```python
from build123d import *

# Parameters (mm, degrees)
SKETCH1_W                      = 172.4
SKETCH1_H                      = 192.4
BOSS_EXTRUDE1_DEPTH            = 6.35
CUT_EXTRUDE1_REACH             = 131.326
SKETCH2_W                      = 41
SKETCH2_H                      = 41
CBORE_FOR_M4_SHCS1_D           = 4.5
CBORE_FOR_M4_SHCS1_CBORE_D     = 8
CBORE_FOR_M4_SHCS1_CBORE_DEPTH = 4
CUT_EXTRUDE3_REACH             = 131.326
SKETCH5_R                      = 1.2
SKETCH6_R                      = 1.4
CUT_EXTRUDE4_DEPTH             = 4
CUT_EXTRUDE5_REACH             = 131.326
SKETCH7_R                      = 1.35
SKETCH8_R                      = 1.5
CUT_EXTRUDE6_DEPTH             = 5
SKETCH9_W                      = 3
SKETCH9_H                      = 192.4
EXTRUDE_THIN1_DEPTH            = 3
CHAMFER1_SIZE                  = 3
CHAMFER2_SIZE                  = 1
CUT_EXTRUDE8_DEPTH             = 302.265202936
CUT_EXTRUDE8_DEPTH_BACK        = 302.265202936
SKETCH11_W                     = 285.28996188
SKETCH11_H                     = 259.000443209
SKETCH11_W_2                   = 75.460655446
SKETCH11_H_2                   = 65.723796679


with BuildPart() as part:
    # Sketch1 → Boss-Extrude1 (new body)
    with BuildSketch(Plane(origin=(0, 0, 0), x_dir=(1, 0, 0), z_dir=(0, 1, 0))):
        Rectangle(SKETCH1_W, SKETCH1_H)
    extrude(amount=BOSS_EXTRUDE1_DEPTH)

    # Sketch2 → Cut-Extrude1 (cut, up to next)
    with BuildSketch(Plane(origin=(0, 6.35, 0), x_dir=(1, 0, 0), z_dir=(0, 1, 0)), mode=Mode.PRIVATE) as cut_extrude1_sk1:
        with Locations((-65.7, 75.7)):
            Rectangle(SKETCH2_W, SKETCH2_H)
    cut_extrude1_tool1 = extrude(cut_extrude1_sk1.sketch, amount=-CUT_EXTRUDE1_REACH, mode=Mode.PRIVATE) & part.part
    add(cut_extrude1_tool1.solids().sort_by_distance((-65.7, 6.35, -75.7))[0], mode=Mode.SUBTRACT)

    # CBORE for M4 SHCS1 (through all)
    with Locations(Plane(origin=(0, 6.35, 0), x_dir=(1, 0, 0), z_dir=(0, 1, 0))):
        with Locations((66.2, 76.2), (-66.2, 34.39549116), (-66.2, -56.2), (-26.2, 76.2)):
            CounterBoreHole(CBORE_FOR_M4_SHCS1_D / 2, CBORE_FOR_M4_SHCS1_CBORE_D / 2, CBORE_FOR_M4_SHCS1_CBORE_DEPTH)

    # Sketch5 → Cut-Extrude3 (cut, up to next)
    with BuildSketch(Plane(origin=(0, 6.35, 0), x_dir=(1, 0, 0), z_dir=(0, 1, 0)), mode=Mode.PRIVATE) as cut_extrude3_sk1:
        with Locations(Location((-76.36, -87.31, 0), (0, 0, 270))):
            Circle(SKETCH5_R)
    cut_extrude3_tool1 = extrude(cut_extrude3_sk1.sketch, amount=-CUT_EXTRUDE3_REACH, mode=Mode.PRIVATE) & part.part
    # Sketch5 → Cut-Extrude3 (cut, up to next)
    with BuildSketch(Plane(origin=(0, 6.35, 0), x_dir=(1, 0, 0), z_dir=(0, 1, 0)), mode=Mode.PRIVATE) as cut_extrude3_sk2:
        with Locations(Location((-56.04, -87.31, 0), (0, 0, 270))):
            Circle(SKETCH5_R)
    cut_extrude3_tool2 = extrude(cut_extrude3_sk2.sketch, amount=-CUT_EXTRUDE3_REACH, mode=Mode.PRIVATE) & part.part
    add(cut_extrude3_tool1.solids().sort_by_distance((-76.36, 6.35, 87.31))[0], mode=Mode.SUBTRACT)
    add(cut_extrude3_tool2.solids().sort_by_distance((-56.04, 6.35, 87.31))[0], mode=Mode.SUBTRACT)

    # Sketch6 → Cut-Extrude4 (cut)
    with BuildSketch(Plane(origin=(0, 6.35, 0), x_dir=(1, 0, 0), z_dir=(0, 1, 0))):
        with Locations(Location((-76.36, -87.31, 0), (0, 0, 270))):
            Circle(SKETCH6_R)
        with Locations(Location((-56.04, -87.31, 0), (0, 0, 270))):
            Circle(SKETCH6_R)
    extrude(amount=-CUT_EXTRUDE4_DEPTH, mode=Mode.SUBTRACT)

    # Sketch7 → Cut-Extrude5 (cut, up to next)
    with BuildSketch(Plane(origin=(0, 6.35, 0), x_dir=(1, 0, 0), z_dir=(0, 1, 0)), mode=Mode.PRIVATE) as cut_extrude5_sk1:
        with Locations(Location((-35.24, -50.96, 0), (0, 0, 270))):
            Circle(SKETCH7_R)
    cut_extrude5_tool1 = extrude(cut_extrude5_sk1.sketch, amount=-CUT_EXTRUDE5_REACH, mode=Mode.PRIVATE) & part.part
    # Sketch7 → Cut-Extrude5 (cut, up to next)
    with BuildSketch(Plane(origin=(0, 6.35, 0), x_dir=(1, 0, 0), z_dir=(0, 1, 0)), mode=Mode.PRIVATE) as cut_extrude5_sk2:
        with Locations(Location((23.46, -50.96, 0), (0, 0, 270))):
            Circle(SKETCH7_R)
    cut_extrude5_tool2 = extrude(cut_extrude5_sk2.sketch, amount=-CUT_EXTRUDE5_REACH, mode=Mode.PRIVATE) & part.part
    add(cut_extrude5_tool1.solids().sort_by_distance((-35.24, 6.35, 50.96))[0], mode=Mode.SUBTRACT)
    add(cut_extrude5_tool2.solids().sort_by_distance((23.46, 6.35, 50.96))[0], mode=Mode.SUBTRACT)

    # Sketch8 → Cut-Extrude6 (cut)
    with BuildSketch(Plane(origin=(0, 6.35, 0), x_dir=(1, 0, 0), z_dir=(0, 1, 0))):
        with Locations(Location((-35.24, -50.96, 0), (0, 0, 270))):
            Circle(SKETCH8_R)
        with Locations(Location((23.46, -50.96, 0), (0, 0, 270))):
            Circle(SKETCH8_R)
    extrude(amount=-CUT_EXTRUDE6_DEPTH, mode=Mode.SUBTRACT)

    # Sketch9 → Extrude-Thin1 (add)
    with BuildSketch(Plane(origin=(0, 6.35, 0), x_dir=(1, 0, 0), z_dir=(0, 1, 0))):
        with Locations((78.7, 0)):
            Rectangle(SKETCH9_W, SKETCH9_H)
    extrude(amount=EXTRUDE_THIN1_DEPTH)

    # Chamfer1
    chamfer1_edges = [part.edges().sort_by_distance(p)[0] for p in [
        (77.2, 6.35, 0),
        (80.2, 6.35, 0),
    ]]
    chamfer(chamfer1_edges, length=CHAMFER1_SIZE - 0.0001)  # a hair under: the kernel refuses the full size

    # Chamfer2
    chamfer2_edges = [part.edges().sort_by_distance(p)[0] for p in [
        (0, 0, 96.2),
        (86.2, 0, 0),
    ]]
    chamfer(chamfer2_edges, length=CHAMFER2_SIZE)


with BuildPart() as body_2:
    # Mirror1: mirrored copy
    add(part.part.mirror(Plane(origin=(1.506427127, 3.750129783, 96.2), x_dir=(1, 0, 0), z_dir=(0, 0, 1))))

    # Sketch11 → Cut-Extrude8 (cut, two sides: drawn at the far end of the back side and taken through both)
    with BuildSketch(Plane(origin=(0, 6.35, 0), x_dir=(1, 0, 0), z_dir=(0, 1, 0)).offset(-CUT_EXTRUDE8_DEPTH_BACK)):
        with Locations((10.467123175, -184.853934456)):
            Rectangle(SKETCH11_W, SKETCH11_H)
        with Locations((-5.84211526, -117.426187493)):
            Rectangle(SKETCH11_W_2, SKETCH11_H_2, mode=Mode.SUBTRACT)
    extrude(amount=CUT_EXTRUDE8_DEPTH + CUT_EXTRUDE8_DEPTH_BACK, mode=Mode.SUBTRACT)


solid = body_2.part
```
Input: part model. Units: mm. Frame: model coordinates. A direction names the side the tool comes from. Coordinates: 2 decimals unless noted, no trailing zeros. Write each loop counter-clockwise with the first axis right and the second up, starting at its lowest first coordinate (ties: lowest second). Pieces come first, ordered by that corner, then holes. Notation, with made-up numbers: (53, 42.25) -> (92, 42.25) arc R10 cw to (92, 55.25) -> close; hole circle Ø10 at (8.5, -31). An arc over 180 degrees is marked (long way). Write each question's results on one line, items separated by ' | '.
Item 1: Material intervals for probe 1 along X at (y, z) = (4.5, 141.5); probe 2 along Z at (x, y) = (11.5, 0.5), sorted ascending.
Conclusion:
probe 1: x = -43.57 to -36.74, -33.74 to 21.96, 24.96 to 31.89 | probe 2: z = 96.7 to 150.29
Item 2: Section query B-B on z = 141.44. Return loops of the section in (x, y).
Conclusion:
outline: (-43.57, 0) -> (-36.59, 0) -> (-36.59, 1.35) -> (-36.74, 1.35) -> (-36.74, 6.35) -> (-43.57, 6.35) -> close; (-33.89, 0) -> (22.11, 0) -> (22.11, 1.35) -> (21.96, 1.35) -> (21.96, 6.35) -> (-33.74, 6.35) -> (-33.74, 1.35) -> (-33.89, 1.35) -> close; (24.81, 0) -> (31.89, 0) -> (31.89, 6.35) -> (24.96, 6.35) -> (24.96, 1.35) -> (24.81, 1.35) -> close
Item 3: Set-up query: faces 1 (the cylindrical face through (22.885, 3.885, 140.054)), 2 (the cylindrical face through (22.943, 0.684, 140.193)). Return all of +Z, -Z, +X, -X, +Y, -Y with unobstructed straight access to the full face (end or side cutting, diameter ignored); none if empty.
Conclusion:
face 1: +Y | face 2: +Y, -Y
Item 4: Pin query (flat end, axial travel): pin 1 Ø1.8 at (x, z) = (23.46, 141.44) entering from -Y; pin 2 Ø3 at (x, z) = (-19, 111.5) entering from -Y. Return the tip coordinate at first contact, or that it passes through.
Conclusion:
pin 1: passes through | pin 2: stops at y = 0
Item 5: Mould query, pull axis X, two halves, no side actions, for faces 3 (the flat face through (-6, 0, 124)), 4 (the cylindrical face through (-34.79, 3.88, 140.01)), 5 (the flat face through (-43.572, 3, 124)), 6 (the flat face through (31.888, 3, 124)). Classes: +X half, -X half, draft (parallel to the pull), parting line (faces both ways), or undercut.
Conclusion:
face 3: draft | face 4: undercut | face 5: -X half | face 6: +X half
Item 6: Section query A-A on x = -35.24. Return loops of the section in (y, z), plus the area to 3 significant figures.
Conclusion:
outline: (0, 97.2) -> (1, 96.2) -> (6.35, 96.2) -> (6.35, 139.94) -> (1.35, 139.94) -> (1.35, 140.09) -> (0, 140.09) -> close; (0, 142.79) -> (1.35, 142.79) -> (1.35, 142.94) -> (6.35, 142.94) -> (6.35, 150.29) -> (0, 150.29) -> close | area: 324 mm^2
